Source: CAD feature listing. Evaluate the final solid. Frame: model axes, mm. Face numbers are marked on the shaded views. A direction names the side the tool comes from. Give positions to 0.01 mm unless a question says otherwise; leave off trailing zeros. Loops run counter-clockwise (first coordinate to the right, second up) from the corner with the lowest first, then second, coordinate; pieces in that order, holes last.
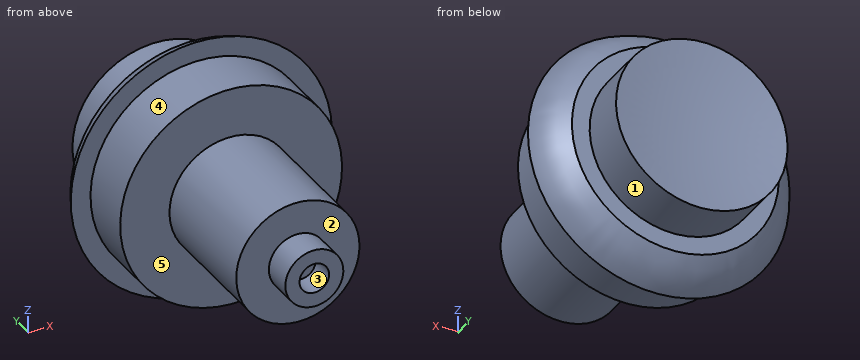
from build123d import *

# Parameters (mm, degrees)
SKETCH2_R          = 1.905
CUT_EXTRUDE1_DEPTH = 3.3782


with BuildPart() as part:
    # Sketch1 → Revolve1 (revolve)
    with BuildSketch(Plane.XY, mode=Mode.PRIVATE) as revolve1_sk:
        with BuildLine():
            Line((0, 0), (0, 37.592))
            ThreePointArc((0, 37.592), (5.560874504, 37.910541815), (11.049, 38.862))
            Line((11.049, 38.862), (11.049, 32.2961))
            Line((11.049, 32.2961), (13.335, 32.2961))
            ThreePointArc((13.335, 32.2961), (15.452618981, 30.510074151), (16.8275, 28.1051))
            Line((16.8275, 28.1051), (14.2875, 28.1051))
            Line((14.2875, 28.1051), (14.2875, 20.7137))
            Line((14.2875, 20.7137), (7.9375, 20.7137))
            Line((7.9375, 20.7137), (7.9375, 4.1021))
            Line((7.9375, 4.1021), (3.7338, 4.1021))
            Line((3.7338, 4.1021), (3.7338, 0))
            Line((3.7338, 0), (0, 0))
        make_face()
    revolve(revolve1_sk.sketch.rotate(Axis((0, 0, 0), (0, 1, 0)), 90), axis=Axis((0, 0, 0), (0, 1, 0)))

    # Sketch2 → Cut-Extrude1 (cut)
    with BuildSketch(Plane.XZ):
        with Locations(Location((0, 0, 0), (0, 0, 270))):
            Circle(SKETCH2_R)
    extrude(amount=-CUT_EXTRUDE1_DEPTH, mode=Mode.SUBTRACT)


solid = part.part
1) Cut plane C-C (y = 5). Return loops of the section in (x, z) (1 decimal), and give its area (3 significant figures).
Checks:
outline: circle Ø15.9 at (0, 0)
area: 198 mm2
2) Ray query, probe 1 along X at (y, z) = (2, 0) (3 decimals); probe 2 along Y at (x, z) = (10.5, 11); probe 3 along Y at (x, z) = (15, 5). Return the intervals inside material, ascending.
Checks:
probe 1: x = -3.734 to -1.905, 1.905 to 3.734
probe 2: y = 28.11 to 30.79
probe 3: y = 28.11 to 30.05
3) Cut plane A-A (x = 0). Return loops of the section in (y, z) (1 decimal), and give its area (3 significant figures).
Checks:
outline: (0, -3.7) - (4.1, -3.7) - (4.1, -7.9) - (20.7, -7.9) - (20.7, -14.3) - (28.1, -14.3) - (28.1, -16.8) arc R7.9 ccw to (32.3, -13.3) - (32.3, -11) - (38.9, -11) arc R48.7 cw to (38.9, 11) - (32.3, 11) - (32.3, 13.3) arc R7.9 ccw to (28.1, 16.8) - (28.1, 14.3) - (20.7, 14.3) - (20.7, 7.9) - (4.1, 7.9) - (4.1, 3.7) - (0, 3.7) - (0, 1.9) - (3.4, 1.9) - (3.4, -1.9) - (0, -1.9) - close
area: 749 mm2
4) Pull-direction query (Z, two-part tool) for the marked faces 3, 4 and 5; classes: released by +Z, released by -Z, zero draft, split by the parting line, or undercut.
Checks:
face 3: undercut
face 4: split by the parting line
face 5: zero draft
5) Reachability of the marked faces 1 and 2 from +Z, -Z, +X, -X, +Y, -Y: full face, straight path, thin tool, end or side. Return the list, or none.
Checks:
face 1: +Y
face 2: -Y
6) Contact query for flat-ended pins moving along their axis: P1, Ø2, axis at y = 7, z = 4, coming from the -X side; P2, Ø1, axis at x = 0, y = 33.5, coming from the +Z side; P3, Ø4, axis at x = -5, z = -8.5, coming from the -Y side; P4, Ø5, axis at y = 16, z = 10.5, coming from the +X side. Output: stop coordinate, or through.
Checks:
P1: stops at x = -7.35
P2: stops at z = 11.05
P3: stops at y = 4.1
P4: passes through
7) Cut plane B-B (z = 0). Return loops of the section in (x, y) (1 decimal), and give its area (3 significant figures).
Checks:
outline: (-16.8, 28.1) - (-14.3, 28.1) - (-14.3, 20.7) - (-7.9, 20.7) - (-7.9, 4.1) - (-3.7, 4.1) - (-3.7, 0) - (-1.9, 0) - (-1.9, 3.4) - (1.9, 3.4) - (1.9, 0) - (3.7, 0) - (3.7, 4.1) - (7.9, 4.1) - (7.9, 20.7) - (14.3, 20.7) - (14.3, 28.1) - (16.8, 28.1) arc R7.9 ccw to (13.3, 32.3) - (11, 32.3) - (11, 38.9) arc R48.7 cw to (-11, 38.9) - (-11, 32.3) - (-13.3, 32.3) arc R7.9 ccw to start
area: 749 mm2
